```python
from build123d import *

# Parameters (mm, degrees)
BOSS_EXTRUDE1_DEPTH                             = 12
FILLET1_R                                       = 10
M5X0_8_TAPPED_HOLE1_D                           = 4.2
M5X0_8_TAPPED_HOLE1_DEPTH                       = 14
M5X0_8_TAPPED_HOLE1_TIP                         = 1.2618073
CBORE_FOR_M5_SOCKET_HEAD_CAP_SCREW1_D           = 5.5
CBORE_FOR_M5_SOCKET_HEAD_CAP_SCREW1_CBORE_D     = 10
CBORE_FOR_M5_SOCKET_HEAD_CAP_SCREW1_CBORE_DEPTH = 5


with BuildPart() as part:
    # Sketch1 → Boss-Extrude1 (new body)
    with BuildSketch(Plane(origin=(0, 0, 0), x_dir=(0, 0, -1), z_dir=(1, 0, 0))):
        Polygon((0, 0), (197.5, 0), (197.5, -75), (20, -75), (20, -100), (0, -100), align=None)
    extrude(amount=BOSS_EXTRUDE1_DEPTH)

    # Fillet1
    fillet1_edges = [part.edges().sort_by_distance(p)[0] for p in [
        (6, -75, -20),
    ]]
    fillet(fillet1_edges, radius=FILLET1_R)

    # M5x0.8 Tapped Hole1
    with Locations(Plane.XY):
        with Locations((6, -6), (6, -50), (6, -94)):
            Hole(M5X0_8_TAPPED_HOLE1_D / 2, depth=M5X0_8_TAPPED_HOLE1_DEPTH)
            with Locations((0, 0, -(M5X0_8_TAPPED_HOLE1_DEPTH + M5X0_8_TAPPED_HOLE1_TIP / 2))):  # 118° drill point
                Cone(0, M5X0_8_TAPPED_HOLE1_D / 2, M5X0_8_TAPPED_HOLE1_TIP, mode=Mode.SUBTRACT)

    # CBORE for M5 Socket Head Cap Screw1 (through all)
    with Locations(Plane(origin=(12, 0, 0), x_dir=(0, 0, -1), z_dir=(1, 0, 0))):
        with Locations((123, -14), (123, -64), (187, -64), (187, -14)):
            CounterBoreHole(CBORE_FOR_M5_SOCKET_HEAD_CAP_SCREW1_D / 2, CBORE_FOR_M5_SOCKET_HEAD_CAP_SCREW1_CBORE_D / 2, CBORE_FOR_M5_SOCKET_HEAD_CAP_SCREW1_CBORE_DEPTH)


solid = part.part
```
Input: part model. Units: mm. Frame: model coordinates. A direction names the side the tool comes from. Round coordinates to 2 decimals unless told otherwise and drop trailing zeros. Order: outer loops, then holes, each group sorted by start corner. A loop starts at its lowest first (then second) coordinate and runs counter-clockwise, first axis right, second up. Notation, with made-up numbers: (15.25, 43.25) - (35.25, 43.25) arc R25 ccw to (35.25, 81.25) - close; hole circle Ø7 at (57.5, 34.25). An arc over 180 degrees is marked (long way). One line per question, with ' | ' between items. Start each with the question number.
1) Ray query, probe 1 along Y at (x, z) = (9.35, -123); probe 2 along Y at (x, z) = (6, -3.25); probe 3 along Y at (x, z) = (3.25, -123). Return the intervals inside material, ascending.
2) Set-up query: faces 4 (the cylindrical face through (10, -61, -183)), 5 (the cylindrical face through (6.46, -52.05, -7.1)), 6 (the flat face through (6, -75, -115)), 7 (the cylindrical face through (3.45, -13.17, -120.38)). Return all of +Z, -Z, +X, -X, +Y, -Y with unobstructed straight access to the full face (end or side cutting, diameter ignored); none if empty.
3) Contact query for flat-ended pins moving along their axis: P1, Ø8, axis at y = -64, z = -123, coming from the +X side; P2, Ø3.5, axis at x = 6, y = -50, coming from the +Z side; P3, Ø1.5, axis at x = 10.5, z = -39, coming from the -Y side. Output: stop coordinate, or through.
4) Cut plane C-C, the plane z = -95.5. Return the cut outline in (x, y), then the cut area to 3 significant figures.
5) Cut plane B-B, the plane z = -187. Return the cut outline in (x, y), then the cut area to 3 significant figures.
6) Pull-direction query (Z, two-part tool) for faces 1 (the flat face through (0, -38, -100)), 2 (the flat face through (3, -51, 0)), 3 (the cylindrical face through (3.45, -13.17, -184.38)); classes: +Z half, -Z half, draft (parallel to the pull), parting line (faces both ways), or undercut.
7) Cut plane A-A, the plane y = -14. Return the cut outline in (x, z).
Worked out:
1) probe 1: y = -75 to -69, -59 to -19, -9 to 0 | probe 2: y = -100 to -96.1, -91.9 to -52.1, -47.9 to -8.1, -3.9 to 0 | probe 3: y = -75 to -66.75, -61.25 to -16.75, -11.25 to 0
2) face 4: +X | face 5: +Z | face 6: -Z, +X, -X, -Y | face 7: +X, -X
3) P1: stops at x = 7 | P2: stops at z = -14.21 | P3: stops at y = -75
4) outline: (0, -75) - (12, -75) - (12, 0) - (0, 0) - close | area: 900 mm^2
5) outline: (0, -75) - (12, -75) - (12, -69) - (7, -69) - (7, -66.75) - (0, -66.75) - close; (0, -61.25) - (7, -61.25) - (7, -59) - (12, -59) - (12, -19) - (7, -19) - (7, -16.75) - (0, -16.75) - close; (0, -11.25) - (7, -11.25) - (7, -9) - (12, -9) - (12, 0) - (0, 0) - close | area: 723 mm^2
6) face 1: draft | face 2: +Z half | face 3: undercut
7) outline: (0, -197.5) - (12, -197.5) - (12, -192) - (7, -192) - (7, -189.75) - (0, -189.75) - close; (0, -184.25) - (7, -184.25) - (7, -182) - (12, -182) - (12, -128) - (7, -128) - (7, -125.75) - (0, -125.75) - close; (0, -120.25) - (7, -120.25) - (7, -118) - (12, -118) - (12, 0) - (0, 0) - close
